Can you work these out from the model? Positions are in its coordinate system, mm. Face numbers are marked on the shaded views. A direction names the side the tool comes from. Round coordinates to 2 decimals unless told otherwise and drop trailing zeros. Order: outer loops, then holes, each group sorted by start corner. A loop starts at its lowest first (then second) coordinate and runs counter-clockwise, first axis right, second up. Notation, with made-up numbers: (-10, 42.25) -> (21, 42.25) arc R20 cw to (21, 73.25) -> close; hole circle Ø8 at (-32.75, 30). An arc over 180 degrees is marked (long way). Use a Markdown table: item, result. Add a question column.
Q1. If we section it at C-C on x = -15: List the corners of the cut face in (y, z) for me.
Q2. If we section it at B-B on y = -23: List the corners of the cut face in (x, z) for me.
Q3. I'm going to push flat-ended pins straight in: pin 1 Ø6 at (x, y) = (-3, -29) entering from -Z; pin 2 Ø6 at (y, z) = (-27.5, -16.5) entering from +X; pin 3 Ø12 at (x, y) = (10.5, -30.5) entering from +Z. Where does each tip first touch, or does it pass through?
Q4. I need wall thicknesses on line 1 along Z through (x, y) = (-15, -1.45); line 2 along X through (y, z) = (-1, 19); line 3 along Z through (x, y) = (26, -14). Which ranges of each line are inside material? Lowest first, please. Write a range as [from, to].
Q5. For the marked faces 1, 2 and 3, which set-ups out of +Z, -Z, +X, -X, +Y, -Y let a thin tool reach every point of the face, with its end or its side?
Q6. If we section it at D-D on z = 19.5: List the corners of the cut face in (x, y) for me, plus the area to 3 significant figures.
Q7. If we section it at A-A on z = 0: List the corners of the cut face in (x, y) for me.
```python
from build123d import *

# Parameters (mm, degrees)
F0_R     = 2
F1_DEPTH = 2
F2_W     = 60
F2_H     = 32
F3_DEPTH = 36
F4_R     = 2
F5_DEPTH = 20


with BuildPart() as f1:
    # F0 (on Front) → F1 (new body)
    with BuildSketch(Plane.XZ):
        with BuildLine():
            ThreePointArc((30, 21.5), (29.414214, 22.914214), (28, 23.5))
            Line((28, 23.5), (-28, 23.5))
            ThreePointArc((-28, 23.5), (-29.414214, 22.914214), (-30, 21.5))
            Line((-30, 21.5), (-30, -21.5))
            ThreePointArc((-30, -21.5), (-29.414214, -22.914214), (-28, -23.5))
            Line((-28, -23.5), (28, -23.5))
            ThreePointArc((28, -23.5), (29.414214, -22.914214), (30, -21.5))
            Line((30, -21.5), (30, 21.5))
        make_face()
        with Locations((-15, -19.5)):
            Circle(F0_R, mode=Mode.SUBTRACT)
        with Locations((15, -19.5)):
            Circle(F0_R, mode=Mode.SUBTRACT)
        with Locations((-15, 19.5)):
            Circle(F0_R, mode=Mode.SUBTRACT)
        with Locations((15, 19.5)):
            Circle(F0_R, mode=Mode.SUBTRACT)
    extrude(amount=F1_DEPTH)

    # F2 (on Front) → F3 (join)
    with BuildSketch(Plane.XZ):
        Rectangle(F2_W, F2_H)
    extrude(amount=F3_DEPTH)

    # F4 (on face) → F5 (join)
    with BuildSketch(Plane.YZ.offset(30)):
        with Locations((-23, 0)):
            Circle(F4_R)
    extrude(amount=F5_DEPTH)


solid = f1.part
```
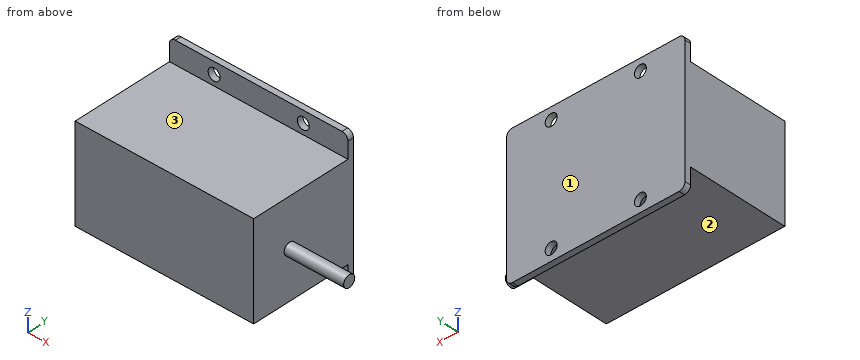
Answer below:
| question | item | result |
|---|---|---|
| 1 | outline | (-36, -16) -> (-2, -16) -> (-2, -17.5) -> (0, -17.5) -> (0, 17.5) -> (-2, 17.5) -> (-2, 16) -> (-36, 16) -> close; (-2, -23.5) -> (0, -23.5) -> (0, -21.5) -> (-2, -21.5) -> close; (-2, 21.5) -> (0, 21.5) -> (0, 23.5) -> (-2, 23.5) -> close |
| 2 | outline | (-30, -16) -> (30, -16) -> (30, -2) -> (50, -2) -> (50, 2) -> (30, 2) -> (30, 16) -> (-30, 16) -> close |
| 3 | pin 1 | z = -16 |
| 3 | pin 2 | x = 30 |
| 3 | pin 3 | z = 16 |
| 4 | line 1 | [-23.5, -21.5], [-17.5, 17.5], [21.5, 23.5] |
| 4 | line 2 | [-30, -16.94], [-13.06, 13.06], [16.94, 30] |
| 4 | line 3 | [-16, 16] |
| 5 | face 1 | +Z, -Z, +X, -X, +Y |
| 5 | face 2 | -Z, +X, -X, -Y |
| 5 | face 3 | +Z, +X, -X, -Y |
| 6 | outline | (-30, -2) -> (-17, -2) -> (-17, 0) -> (-30, 0) -> close; (-13, -2) -> (13, -2) -> (13, 0) -> (-13, 0) -> close; (17, -2) -> (30, -2) -> (30, 0) -> (17, 0) -> close |
| 6 | area | 104 mm² |
| 7 | outline | (-30, -36) -> (30, -36) -> (30, -25) -> (50, -25) -> (50, -21) -> (30, -21) -> (30, 0) -> (-30, 0) -> close |
